```python
from build123d import *

# Parameters (mm, degrees)
F0_R          = 19.2057063742
F1_DEPTH      = 30.48
F1_TAPER      = -3
F1_DEPTH_BACK = 30.48
F1_TAPER_BACK = -3
F2_T          = -2.54


# Not quite as in the source:
# - a fillet or chamfer that OpenCascade refuses, or shapes differently, is made with other operations: its cross-section is extruded or revolved along the edge and cut away or added


with BuildPart() as f1:
    # F0 (on Front) → F1 (new body, two sides)
    with BuildSketch(Plane.XZ) as f1_sk:
        Circle(F0_R)
    extrude(amount=F1_DEPTH, taper=F1_TAPER)
    extrude(f1_sk.sketch, amount=-F1_DEPTH_BACK, taper=F1_TAPER_BACK)

    # F2
    f2_openings = [f1.faces().sort_by_distance(p)[0] for p in [
        (0, -30.48, 0),
        (0, 30.48, 0),
    ]]
    offset(amount=F2_T, openings=f2_openings, kind=Kind.INTERSECTION)

    # F3: fillet of radius 2.54 on 3 edges, made by hand

    # F3_s1 → F3_t2 (revolve)
    with BuildSketch(Plane.XY):
        with BuildLine():
            ThreePointArc((19.2126731148, 0.1329333289), (19.2091921331, 0), (19.2126731148, -0.1329333289))
            Line((19.2126731148, -0.1329333289), (19.1619427344, -0.1355919954))
            Line((19.1619427344, -0.1355919954), (19.1548366591, 0))
            Line((19.1548366591, 0), (19.1619427344, 0.1355919954))
            Line((19.1619427344, 0.1355919954), (19.2126731148, 0.1329333289))
        make_face()
    revolve(axis=Axis((0, 0, 0), (0, -1, 0)))

    # F3_s3 → F3_t4 (revolve, cut)
    with BuildSketch(Plane.XY):
        with BuildLine():
            ThreePointArc((20.6631954174, 27.8105476529), (20.0142642558, 29.6430727219), (18.2596097279, 30.48))
            Line((18.2596097279, 30.48), (18.2622683945, 30.5307303804))
            ThreePointArc((18.2622683945, 30.5307303804), (19.5313526074, 30.5308), (20.8030954868, 30.5308))
            Line((20.8030954868, 30.5308), (20.8538258671, 30.4773413334))
            Line((20.8538258671, 30.4773413334), (20.7139257977, 27.8078889863))
            Line((20.7139257977, 27.8078889863), (20.6631954174, 27.8105476529))
        make_face()
    revolve(axis=Axis((0, 30.48, 0), (0, -1, 0)), mode=Mode.SUBTRACT)

    # F3_s5 → F3_t6 (revolve, cut)
    with BuildSketch(Plane.XY):
        with BuildLine():
            ThreePointArc((20.6631954174, -27.8105476529), (20.0142642558, -29.6430727219), (18.2596097279, -30.48))
            Line((18.2596097279, -30.48), (18.2622683945, -30.5307303804))
            ThreePointArc((18.2622683945, -30.5307303804), (19.5313526074, -30.5308), (20.8030954868, -30.5308))
            Line((20.8030954868, -30.5308), (20.8538258671, -30.4773413334))
            Line((20.8538258671, -30.4773413334), (20.7139257977, -27.8078889863))
            Line((20.7139257977, -27.8078889863), (20.6631954174, -27.8105476529))
        make_face()
    revolve(axis=Axis((0, -30.48, 0), (0, 1, 0)), mode=Mode.SUBTRACT)


solid = f1.part
```
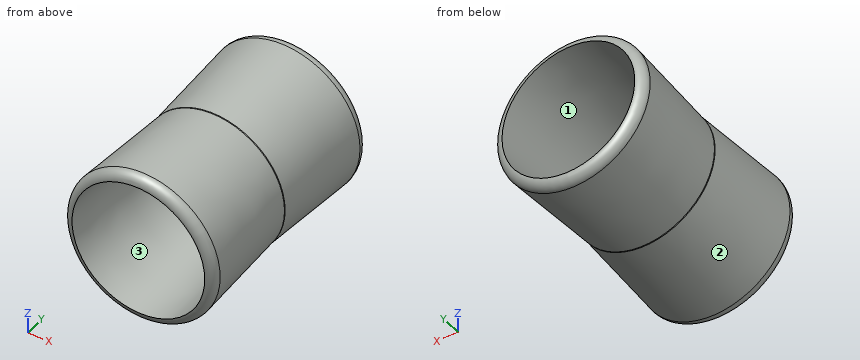
Design review of the part built by this model. Coordinates are the model's own, in mm. Face numbers are marked on the shaded views. Coordinates: 2 decimals unless noted, no trailing zeros. Order: outer loops, then holes, each group sorted by start corner. A loop starts at its lowest first (then second) coordinate and runs counter-clockwise, first axis right, second up. Notation, with made-up numbers: (0, -5.75) - (51, -5.75) arc R26 ccw to (51, 8.25) - close; hole circle Ø7 at (11, -10). An arc over 180 degrees is marked (long way). One line per question, with ' | ' between items.
Q1. Clearance check with flat-ended pins moving along their axes: pin 1 Ø1.5 at (y, z) = (9.5, 9) entering from +X; pin 2 Ø8 at (x, z) = (16, 14.5) entering from +Y; pin 3 Ø4 at (x, y) = (-16.5, 11) entering from +Z; pin 4 Ø10 at (y, z) = (11.5, 3.5) entering from -X. State where each tip first meets the part, or that it passes through.
Answer key:
pin 1: stops at x = 17.9 | pin 2: stops at y = 30.48 | pin 3: stops at z = 13.46 | pin 4: stops at x = -20.01
Q2. Consider section C-C, the plane y = 8. Give the boundary of the cut face in (x, z).
Answer key:
outline: circle Ø39.25 at (0, 0); hole circle Ø34.16 at (0, 0)
Q3. The part is to be moulded in two halves that separate along Y. For the marked faces 1, 2 and 3, say which applies: +Y half, -Y half, draft (parallel to the pull), parting line (faces both ways), or undercut.
Answer key:
face 1: +Y half | face 2: undercut | face 3: -Y half
Q4. To check wall thickness, follow line 1 along X through (y, z) = (-24, 11); line 2 along X through (y, z) = (5, 10); line 3 along Z through (x, y) = (-1, -3). State the ranges of each line that lie inside material, in increasing order.
Answer key:
line 1: x = -17.26 to -14.15, 14.15 to 17.26 | line 2: x = -16.7 to -13.65, 13.65 to 16.7 | line 3: z = -19.34 to -16.79, 16.79 to 19.34
Q5. Consider section B-B, the plane y = -7. Give the boundary of the cut face in (x, z), then the cut area to 3 significant figures.
Answer key:
outline: circle Ø39.15 at (0, 0); hole circle Ø34.06 at (0, 0) | area: 292 mm2
Q6. Consider section A-A, the plane x = 0. Give the boundary of the cut face in (y, z), then the cut area to 3 significant figures.
Answer key:
outline: (-30.48, -18.26) arc R2.54 ccw to (-27.81, -20.66) - (-0.13, -19.21) arc R2.54 cw to (0.13, -19.21) - (27.81, -20.66) arc R2.54 ccw to (30.48, -18.26) - (0, -16.66) - close; (-30.48, 18.26) - (0, 16.66) - (30.48, 18.26) arc R2.54 ccw to (27.81, 20.66) - (0.13, 19.21) arc R2.54 cw to (-0.13, 19.21) - (-27.81, 20.66) arc R2.54 ccw to start | area: 304 mm2
